Input: part model. Units: mm. Frame: model coordinates. A direction names the side the tool comes from. Coordinates: 2 decimals unless noted, no trailing zeros. Order: outer loops, then holes, each group sorted by start corner. A loop starts at its lowest first (then second) coordinate and runs counter-clockwise, first axis right, second up.
from build123d import *

# Parameters (mm, degrees)
SKETCH4_R           = 157.5
SKETCH4_R_2         = 125
BOSS_EXTRUDE1_DEPTH = 135
SKETCH5_W           = 50
SKETCH5_H           = 60
CUT_EXTRUDE1_DEPTH  = 447.397941427
CIRPATTERN1_COUNT   = 12


with BuildPart() as part:
    # Sketch3 → Revolve1 (revolve)
    with BuildSketch(Plane(origin=(0, 0, 0), x_dir=(0, 0, -1), z_dir=(1, 0, 0))):
        Polygon((-212.5, 8.070339729), (-212.5, 35.553232656), (-207.5, 35.553232656), (-207.5, 8.070339729), (0, 8.070339729), (0, -14.446767344), (-207.5, -14.446767344), (-299, -14.446767344), (-299, 8.070339729), (-273.25, 8.070339729), (-273.25, -3.929660271), (-233.25, -3.929660271), (-233.25, 8.070339729), align=None)
    revolve(axis=Axis((0, 120.738006406, 0), (0, -1, 0)))

    # Sketch4 → Boss-Extrude1 (add)
    with BuildSketch(Plane(origin=(0, 8.070339729, 0), x_dir=(1, 0, 0), z_dir=(0, 1, 0))):
        with Locations(Location((0, 0, 0), (0, 0, 270))):
            Circle(SKETCH4_R)
        with Locations(Location((0, 0, 0), (0, 0, 270))):
            Circle(SKETCH4_R_2, mode=Mode.SUBTRACT)
    extrude(amount=BOSS_EXTRUDE1_DEPTH)

    # Sketch5 → Cut-Extrude1 (cut, symmetric)
    with BuildSketch(Plane.XY):
        with Locations((0, 93.070339729)):
            Rectangle(SKETCH5_W, SKETCH5_H)
    cut_extrude1 = extrude(amount=CUT_EXTRUDE1_DEPTH, both=True, mode=Mode.SUBTRACT)

    # CirPattern1: Cut-Extrude1 ×12 about axis
    cirpattern1_axis = Axis((0, 0, 0), (0, 1, 0))
    for i in range(1, CIRPATTERN1_COUNT):
        add(cut_extrude1.rotate(cirpattern1_axis, i * 360 / CIRPATTERN1_COUNT), mode=Mode.SUBTRACT)


solid = part.part
Item 1: Access query for faces 5 (the face through (-107.67, 92.65, 91.03)), 6 (the face through (108.07, 92.65, -91.26)), 7 (the face through (91.26, 92.65, 108.07)). Directions: +Z, -Z, +X, -X, +Y, -Y. A direction counts if a zero-diameter tool reaches every point of the face in a straight line with its end or side. Return the directions, or none.
Response values:
face 5: -X
face 6: +X
face 7: +Z
Item 2: Draft query along Y for faces 1 (the face through (-140.238, 21.619, -152.936)), 2 (the face through (121, 123.07, 70)), 3 (the face through (-91.03, 92.65, 107.67)), 4 (the face through (117, 143.07, -47)). Return one class per face: pulls with the +Y half, pulls with the -Y half, needs draft (parallel to the pull), parting line crosses it, or undercut.
Response values:
face 1: needs draft
face 2: undercut
face 3: undercut
face 4: pulls with the +Y half
Item 3: Cut plane B-B on z = 0. Count the separate pieces of the cut face and the enclosed holes in it, then the cut area to 3 significant figures.
Response values:
separate pieces: 3
enclosed holes: 0
area: 17,700 mm2
Item 4: Cut plane A-A on y = 130.5. Return loops of the section in (x, z), then the cut area to 3 significant figures.
Response values:
outline: circle Ø315 at (0, 0); hole circle Ø250 at (0, 0)
area: 28,800 mm2
Item 5: Pin query (flat end, axial travel): pin 1 Ø16.5 at (y, z) = (88, -146.5) entering from +X; pin 2 Ø1 at (x, z) = (203.5, -123) entering from +Y; pin 3 Ø1 at (x, y) = (-91, 95.5) entering from +Z. Return the tip coordinate at first contact, or that it passes through.
Response values:
pin 1: stops at x = 56.1
pin 2: stops at y = -3.93
pin 3: stops at z = 108.48
Item 6: Ray query, probe 1 along Z at (x, y) = (0, 1.75); probe 2 along X at (y, z) = (22, 0). Return the intervals inside material, ascending.
Response values:
probe 1: z = -299 to -273.25, -233.25 to 233.25, 273.25 to 299
probe 2: x = -212.5 to -207.5, -157.5 to -125, 125 to 157.5, 207.5 to 212.5
